Solid Edge part; units mm, degrees
sketch "Sketch1" plane through (0, 0, 0) normal (0, 0, 1) x (1, 0, 0)
  line L0 (4, -30) -> (4, 30)
  arc A0 (4, 30) -> (1.5199, 33.7) centre (0, 30) ccw
  line L1 (0.5, 60) -> (1.5199, 33.7)
  line L2 (0.5, 60) -> (-1, 62)
  line L3 (-1, 62) -> (2, 64)
  line L4 (2, 64) -> (-1, 66)
  line L5 (-1, 66) -> (2, 68)
  line L6 (2, 68) -> (-1, 70)
  line L7 (-1, 70) -> (2, 72)
  line L8 (2, 72) -> (-1, 74)
  line L9 (-1, 74) -> (2, 76)
  line L10 (2, 76) -> (0.0998, 77.5782)
  arc A1 (-0.2166, 77.2725) -> (0.0998, 77.5782) centre (-0.0407, 77.407) cw
  line L11 (0.75, 76.0085) -> (-0.2166, 77.2725)
  line L12 (-2.25, 74.0085) -> (0.75, 76.0085)
  line L13 (0.75, 72.0085) -> (-2.25, 74.0085)
  line L14 (-2.25, 70.0085) -> (0.75, 72.0085)
  line L15 (0.75, 68.0085) -> (-2.25, 70.0085)
  line L16 (-2.25, 66.0085) -> (0.75, 68.0085)
  line L17 (0.75, 64.0085) -> (-2.25, 66.0085)
  line L18 (-2.25, 62.0085) -> (0.75, 64.0085)
  line L19 (-0.75, 60.0085) -> (-2.25, 62.0085)
  line L20 (-0.75, 60.0085) -> (-1.5199, 33.7)
  arc A2 (-4, 30) -> (-1.5199, 33.7) centre (0, 30) cw
  line L21 (-4, 30) -> (-4, -30)
  arc A3 (-4, -30) -> (4, -30) centre (0, -30) ccw
  dimension "D1" = 4
  dimension "D2" = 0.5
extrude "Ajout_matière_1" add sketch "Sketch1" along normal blind 1
sketch "Sketch2" plane through (0, 0, 0) normal (0, 0, 1) x (1, 0, 0)
  circle A0 centre (0, -30) radius 2
extrude "Cutout1" cut sketch "Sketch2" along normal up to next
fillet "Congé_1" radius 0.5 8 edges at (-2.25, 62.0085, 0.5) (-2.25, 66.0085, 0.5) (-2.25, 70.0085, 0.5) (-2.25, 74.0085, 0.5) (2, 64, 0.5) (2, 68, 0.5) (2, 72, 0.5) (2, 76, 0.5)
fillet "Congé_2" radius 0.5 8 edges at (0.75, 64.0085, 0.5) (0.75, 72.0085, 0.5) (0.75, 68.0085, 0.5) (0.75, 76.0085, 0.5) (-1, 74, 0.5) (-1, 70, 0.5) (-1, 66, 0.5) (-1, 62, 0.5)
properties material "Acier S235"
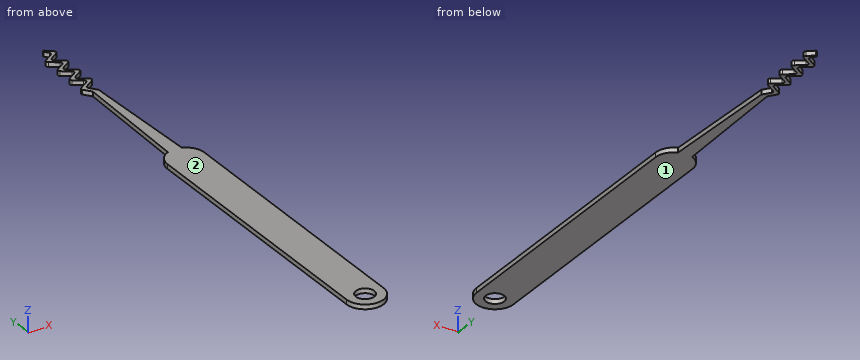
Part model, mm, in its own coordinate system. Face numbers are marked on the shaded views. Coordinates: 2 decimals unless noted, no trailing zeros. Loops run counter-clockwise (first coordinate to the right, second up) from the corner with the lowest first, then second, coordinate; pieces in that order, holes last. Notation, with made-up numbers: (-8.5, -32) - (24.5, -32) arc R7 ccw to (24.5, -27) - close; hole circle Ø11 at (56.25, 62). An arc over 180 degrees is marked (long way). Write each question's results on one line, items separated by ' | '. Start each with the question number.
Q1. Probe line 1 along X through (y, z) = (-30, 0.45); line 2 along X through (y, z) = (69, 0.8); line 3 along X through (y, z) = (62, 0.8). List the from-to ranges inside material, lowest first.
Q2. Drop a flat-ended pin along its axis: pin 1 Ø3 at (x, y) = (-1.5, 14) entering from -Z. Give the stop position or say it passes through.
Q3. Two-plate mould, pull along Z, no slides. Class the marked faces 1 and 2: +Z half, -Z half, draft (parallel to the pull), parting line (faces both ways), or undercut.
Q4. Slice it at A-A on x = -3. Give the cut face in (y, z), and give its area (3 significant figures).
Q5. Slice it at B-B on y = 57. Give the cut face in (x, z).
Answer:
1) line 1: x = -4 to -2, 2 to 4 | line 2: x = -0.74 to 0.5 | line 3: x = -2.02 to -0.77
2) pin 1: stops at z = 0
3) face 1: -Z half | face 2: +Z half
4) outline: (-32.65, 0) - (32.65, 0) - (32.65, 1) - (-32.65, 1) - close | area: 65.3 mm2
5) outline: (-0.84, 0) - (0.62, 0) - (0.62, 1) - (-0.84, 1) - close
